The drawing under review shows one solid part. Ordinate dimensions are in mm from its lowest x, y, z. A direction names the side the tool comes from. Coordinates: 2 decimals unless noted, no trailing zeros. Write each loop counter-clockwise with the first axis right and the second up, starting at its lowest first coordinate (ties: lowest second). Pieces come first, ordered by that corner, then holes.
Q1. Machinability: for the marked faces 1 and 2, which of the approach directions +Z, -Z, +X, -X, +Y, -Y give a long, thin tool a straight path to every point of the face, cutting with its end or side? Answer none if there is none.
Q2. Add section A-A, the plane z = 7.75. Give the boundary of the cut face in (x, y), plus the area to 3 significant figures.
Q3. Add section D-D, the plane x = 11.5. Give the boundary of the cut face in (y, z).
Q4. Clearance check with flat-ended pins moving along their axes: pin 1 Ø3.5 at (x, z) = (20, 7.75) entering from -Y; pin 2 Ø2.5 at (y, z) = (19, 16) entering from -X; pin 3 Ø1 at (x, z) = (34.5, 6.5) entering from +Y; pin 4 Ø3.5 at (x, y) = (19.5, 19) entering from -Z. State where each tip first meets the part, or that it passes through.
Q5. Add section B-B, the plane x = 20. Give the boundary of the cut face in (y, z), plus the area to 3 significant figures.
Q6. Add section C-C, the plane y = 5.75. Give the boundary of the cut face in (x, z) (3 decimals), plus the area to 3 significant figures.
Q7. To check wall thickness, follow probe 1 along X at (y, z) = (7, 0.65); probe 2 along Z at (x, y) = (21, 19.25) (1 decimal); probe 3 along Z at (x, y) = (32, 13.25). State the ranges of each line that lie inside material, in increasing order.
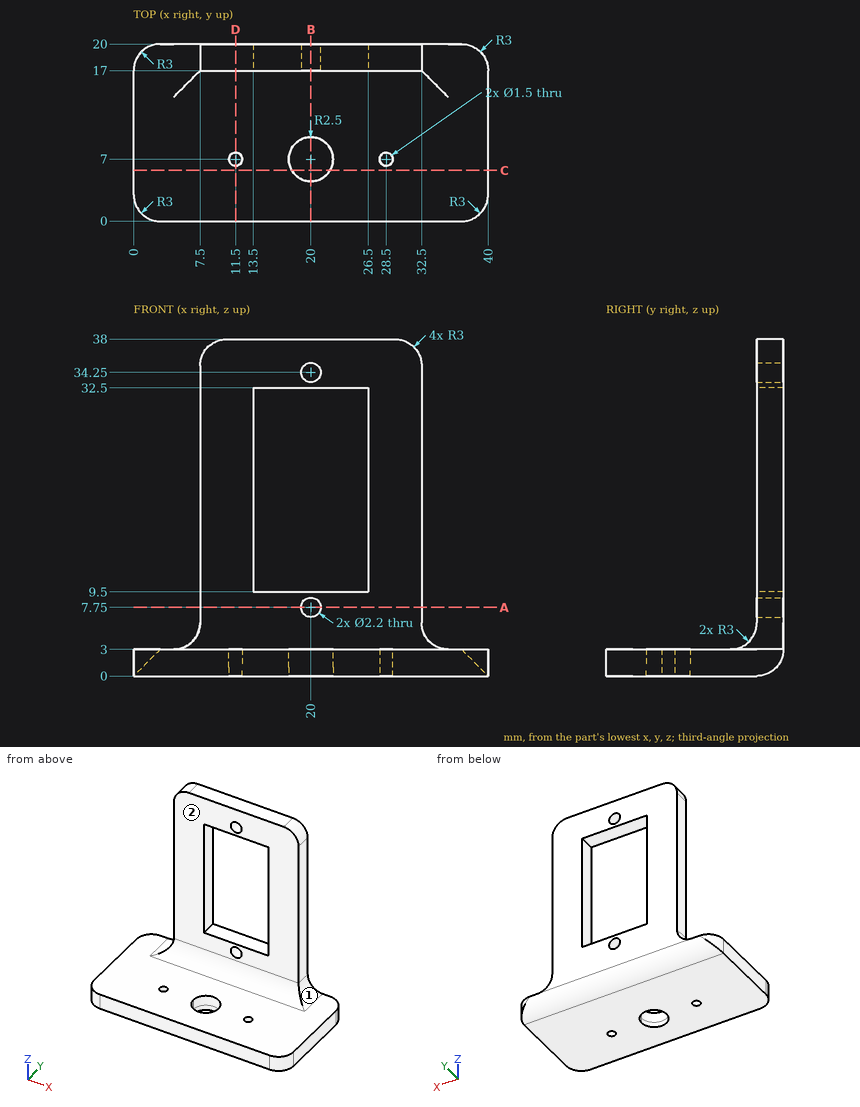
Here are the results:
1. face 1: +Z, +X, +Y, -Y
1. face 2: +Z, +X, -X, -Y
2. outline: (7.5, 17) - (18.9, 17) - (18.9, 20) - (7.5, 20) - close; (21.1, 17) - (32.5, 17) - (32.5, 20) - (21.1, 20) - close
2. area: 68.4 mm2
3. outline: (0, 0) - (6.25, 0) - (6.25, 3) - (0, 3) - close; (7.75, 0) - (17, 0) arc R3 ccw to (20, 3) - (20, 38) - (17, 38) - (17, 6) arc R3 cw to (14, 3) - (7.75, 3) - close
4. pin 1: stops at y = 17
4. pin 2: stops at x = 7.5
4. pin 3: passes through
4. pin 4: stops at z = 0.01
5. outline: (0, 0) - (4.5, 0) - (4.5, 3) - (0, 3) - close; (9.5, 0) - (17, 0) arc R3 ccw to (20, 3) - (20, 6.65) - (17, 6.65) - (17, 6) arc R3 cw to (14, 3) - (9.5, 3) - close; (17, 8.85) - (20, 8.85) - (20, 9.5) - (17, 9.5) - close; (17, 32.5) - (20, 32.5) - (20, 33.15) - (17, 33.15) - close; (17, 35.35) - (20, 35.35) - (20, 38) - (17, 38) - close
5. area: 67.8 mm2
6. outline: (0, 0) - (17.835, 0) - (17.835, 3) - (0, 3) - close; (22.165, 0) - (40, 0) - (40, 3) - (22.165, 3) - close
6. area: 107 mm2
7. probe 1: x = 0 to 10.75, 12.25 to 17.5, 22.5 to 27.75, 29.25 to 40
7. probe 2: z = 1 to 7.3, 8.2 to 9.5, 32.5 to 33.8, 34.7 to 38
7. probe 3: z = 0 to 3
